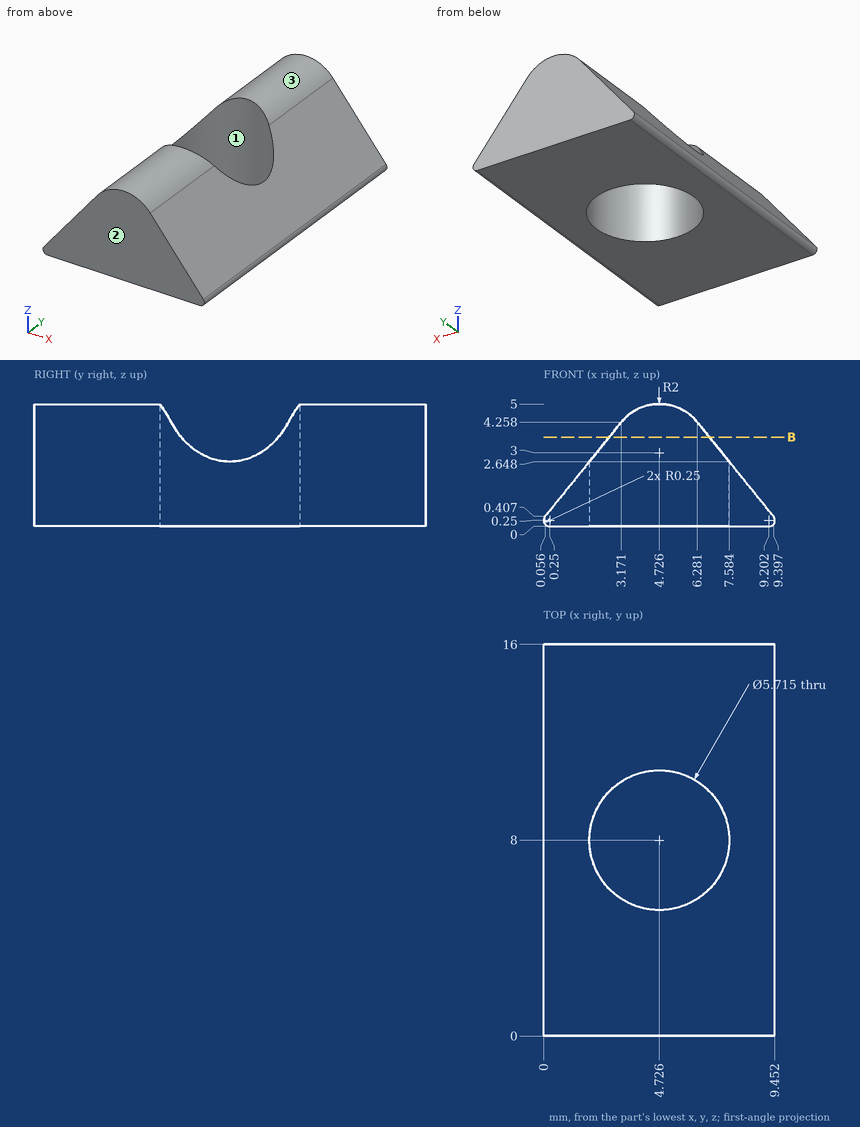
Input: dimensioned drawing with shaded views. Units: mm. Origin: part minimum x, y, z. Coordinates: 2 decimals unless noted, no trailing zeros. Loops run counter-clockwise (first coordinate to the right, second up) from the corner with the lowest first, then second, coordinate; pieces in that order, holes last. Notation, with made-up numbers: M 79.5,-1 L 88.5,-1 A25 ccw 88.5,34 Z; hole C 35,8 d5. An arc over 180 degrees is marked long. One line per item, written item: value. Start each with the question number.
1) Pin query (flat end, axial travel): P1, Ø1.5, axis at x = 1.5, y = 14, coming from the +Z side. Return the tip coordinate at first contact, or that it passes through.
2) Cut plane B-B (z = 3.65). Return loops of the section in (x, y) (1 decimal), then the cut area to 3 significant figures.
3) Material intervals for L1, parallel to Y at x = 4.75, z = 2.9; L2, parallel to Y at x = 6, z = 4.1; L3, parallel to X at y = 10.5, z = 1.4 (1 decimal), sorted ascending. Write a range as from..to.
4) Draft query along X for the marked faces 1, 2 and 3. Return one class per face: released by +X, released by -X, zero draft, split by the parting line, or undercut.
Evaluation:
1. P1: z = 3.12
2. outline: M 2.7,0 L 6.8,0 L 6.8,6 A2.9 cw 2.7,6 Z; M 2.7,10 A2.9 cw 6.8,10 L 6.8,16 L 2.7,16 Z
2. area: 44.3 mm^2
3. L1: 0..5.14, 10.86..16
3. L2: 0..5.44, 10.56..16
3. L3: 0.9..3.3, 6.1..8.6
4. face 1: undercut
4. face 2: zero draft
4. face 3: split by the parting line
